from build123d import *

# Parameters (mm, degrees)
F0_R     = 3.175
F1_DEPTH = 25.4


with BuildPart() as f1:
    # F0 (on Top) → F1 (new body)
    with BuildSketch(Plane.XY):
        with BuildLine():
            ThreePointArc((9.4502929642, 115.490625), (0, 123.825), (-9.4502929642, 115.490625))
            ThreePointArc((-9.4502929642, 115.490625), (-7.14375, 107.9998046905), (0, 104.775))
            ThreePointArc((0, 104.775), (6.7351920908, 107.5648079092), (9.525, 114.3))
            ThreePointArc((9.525, 114.3), (9.5063048942, 114.896483242), (9.4502929642, 115.490625))
        make_face()
        with BuildLine():
            ThreePointArc((3.175, 114.3), (2.2450640303, 112.0549359697), (0, 111.125))
            ThreePointArc((0, 111.125), (-2.2450640303, 116.5450640303), (3.175, 114.3))
        make_face(mode=Mode.SUBTRACT)
        with BuildLine():
            Line((0, 100.0252), (0, 79.375))
            ThreePointArc((0, 79.375), (10.5003255158, 75.40625), (15.7504882737, 65.484375))
            Line((15.7504882737, 65.484375), (9.4502929642, 115.490625))
            ThreePointArc((9.4502929642, 115.490625), (9.5063048942, 114.896483242), (9.525, 114.3))
            ThreePointArc((9.525, 114.3), (6.7351920908, 107.5648079092), (0, 104.775))
            Line((0, 104.775), (0, 100.0252))
        make_face()
        with BuildLine():
            Line((-9.4502929642, 115.490625), (-15.7504882737, 65.484375))
            ThreePointArc((-15.7504882737, 65.484375), (-10.5003255158, 75.40625), (0, 79.375))
            Line((0, 79.375), (0, 100.0252))
            Line((0, 100.0252), (0, 104.775))
            ThreePointArc((0, 104.775), (-7.14375, 107.9998046905), (-9.4502929642, 115.490625))
        make_face()
        with Locations((-3.175, 100.0252)):
            Circle(F0_R, mode=Mode.SUBTRACT)
        with BuildLine():
            ThreePointArc((-9.4772553384, -0.9525), (-7.063929059, 6.3895642457), (0, 9.525))
            Line((0, 9.525), (0, 47.625))
            ThreePointArc((0, 47.625), (-10.6492737428, 51.7267849017), (-15.7954255641, 61.9125))
            Line((-15.7954255641, 61.9125), (-9.4772553384, -0.9525))
        make_face()
        with BuildLine():
            Line((0, 47.625), (0, 9.525))
            ThreePointArc((0, 9.525), (6.7351920908, 6.7351920908), (9.525, 0))
            Line((9.525, 0), (36.5125, 0))
            ThreePointArc((36.5125, 0), (38.9384772185, 5.7120069047), (44.7334821429, 7.9324362036))
            Line((44.7334821429, 7.9324362036), (18.9676000005, 8.8532337108))
            ThreePointArc((18.9676000005, 8.8532337108), (13.2611998974, 11.5713591498), (11.3411865923, 17.5933818124))
            Line((11.3411865923, 17.5933818124), (15.7954255641, 61.9125))
            ThreePointArc((15.7954255641, 61.9125), (10.6492737428, 51.7267849017), (0, 47.625))
        make_face()
        with BuildLine():
            Line((0, 60.325), (0, 47.625))
            ThreePointArc((0, 47.625), (10.6492737428, 51.7267849017), (15.7954255641, 61.9125))
            ThreePointArc((15.7954255641, 61.9125), (15.8550939106, 62.7052534459), (15.875, 63.5))
            ThreePointArc((15.875, 63.5), (15.8438414904, 64.4941387366), (15.7504882737, 65.484375))
            ThreePointArc((15.7504882737, 65.484375), (10.5003255158, 75.40625), (0, 79.375))
            Line((0, 79.375), (0, 66.675))
            ThreePointArc((0, 66.675), (2.2450640303, 65.7450640303), (3.175, 63.5))
            ThreePointArc((3.175, 63.5), (2.2450640303, 61.2549359697), (0, 60.325))
        make_face()
        with BuildLine():
            ThreePointArc((-15.7954255641, 61.9125), (-10.6492737428, 51.7267849017), (0, 47.625))
            Line((0, 47.625), (0, 60.325))
            ThreePointArc((0, 60.325), (-3.175, 63.5), (0, 66.675))
            Line((0, 66.675), (0, 79.375))
            ThreePointArc((0, 79.375), (-10.5003255158, 75.40625), (-15.7504882737, 65.484375))
            ThreePointArc((-15.7504882737, 65.484375), (-15.8737438155, 63.6997054867), (-15.7954255641, 61.9125))
        make_face()
        with BuildLine():
            Line((0, 9.525), (0, 3.175))
            ThreePointArc((0, 3.175), (2.2450640303, 2.2450640303), (3.175, 0))
            Line((3.175, 0), (9.525, 0))
            ThreePointArc((9.525, 0), (6.7351920908, 6.7351920908), (0, 9.525))
        make_face()
        with BuildLine():
            ThreePointArc((3.175, 0), (-2.2450640303, -2.2450640303), (0, 3.175))
            Line((0, 3.175), (0, 9.525))
            ThreePointArc((0, 9.525), (-7.063929059, 6.3895642457), (-9.4772553384, -0.9525))
            ThreePointArc((-9.4772553384, -0.9525), (-6.2623833816, -7.1769199091), (0.3401785714, -9.5189234444))
            ThreePointArc((0.3401785714, -9.5189234444), (6.8544082857, -6.6138273378), (9.525, 0))
            Line((9.525, 0), (3.175, 0))
        make_face()
        with BuildLine():
            Line((36.5125, 0), (9.525, 0))
            ThreePointArc((9.525, 0), (6.8544082857, -6.6138273378), (0.3401785714, -9.5189234444))
            Line((0.3401785714, -9.5189234444), (44.7334821429, -7.9324362036))
            ThreePointArc((44.7334821429, -7.9324362036), (38.9384772185, -5.7120069047), (36.5125, 0))
        make_face()
        with BuildLine():
            ThreePointArc((44.7334821429, 7.9324362036), (38.9384772185, 5.7120069047), (36.5125, 0))
            ThreePointArc((36.5125, 0), (38.9384772185, -5.7120069047), (44.7334821429, -7.9324362036))
            ThreePointArc((44.7334821429, -7.9324362036), (50.1620069047, -5.5115227815), (52.3875, 0))
            ThreePointArc((52.3875, 0), (50.1620069047, 5.5115227815), (44.7334821429, 7.9324362036))
        make_face()
        with BuildLine():
            ThreePointArc((47.625, 0), (44.45, -3.175), (41.275, 0))
            ThreePointArc((41.275, 0), (44.45, 3.175), (47.625, 0))
        make_face(mode=Mode.SUBTRACT)
    extrude(amount=F1_DEPTH)


solid = f1.part
Part model, mm, in its own coordinate system. A direction names the side the tool comes from. Coordinates: 2 decimals unless noted, no trailing zeros. Loops run counter-clockwise (first coordinate to the right, second up) from the corner with the lowest first, then second, coordinate; pieces in that order, holes last. Notation, with made-up numbers: (63, -16.5) -> (116, -16.5) arc R4 cw to (116, -9.5) -> close; hole circle Ø5 at (8.5, -39). An arc over 180 degrees is marked (long way). Use a Markdown table: item, result. Add a question column.
Item 1: Pull direction X, two halves, no side cores. Call faces 3 (the cylindrical face through (-3.588, 103.173, 12.522)), 4 (the cylindrical face through (41.52, -1.22, 12.52)), 5 (the cylindrical face through (-15.873, 63.725, 12.522)), 6 (the cylindrical face through (13.321, 11.503, 12.522)): +X half, -X half, draft (parallel to the pull), parting line (faces both ways), or undercut.
Item 2: Probe probe 1 along Y at (x, z) = (44.45, 10.75) (3 decimals); probe 2 along Y at (x, z) = (-4, 12); probe 3 along Y at (x, z) = (28.5, 2.75). List the from-to ranges inside material, lowest first.
Item 3: Flat gauge pins, fed straight in: P1, Ø5, axis at x = 22.5, z = 9.5, coming from the +Y side; P2, Ø6, axis at x = 1, z = 15.5, coming from the -Y side (3 decimals); P3, Ø1.5, axis at x = -7, z = 12.5, coming from the +Y side; P4, Ø3, axis at x = 24.5, z = 11, coming from the -Y side. Where does each tip first touch, or does it go through?
Item 4: Which spindle directions (+Z, -Z, +X, -X, +Y, -Y) get a long thin tool onto all of the face, cutting with end or side? Do faces 1 (the flat face through (13.537, 39.443, 12.522)), 2 (the flat face through (-12.68, 30.92, 12.52)). Say none if no direction does.
Item 5: Band-saw the part on C-C on y = 86.5. Write the cut outline in (x, z), plus the area to 3 significant figures.
Item 6: Band-saw the part on D-D on x = 7. Write the cut outline in (y, z).
Item 7: Band-saw the part on A-A on x = -1.5. Write the cut outline in (y, z).
Item 8: Band-saw the part on B-B on z = 2.5. Give the number of separate pieces and of enclosed holes in the cut face, plus the area to 3 significant figures.
Geometry says:
| question | item | result |
|---|---|---|
| 1 | face 3 | undercut |
| 1 | face 4 | undercut |
| 1 | face 5 | -X half |
| 1 | face 6 | +X half |
| 2 | probe 1 | -7.943 to -3.175, 3.175 to 7.943 |
| 2 | probe 2 | -8.64 to 96.96, 103.09 to 122.94 |
| 2 | probe 3 | -8.51 to 8.51 |
| 3 | P1 | y = 8.82 |
| 3 | P2 | y = -9.525 |
| 3 | P3 | y = 121.49 |
| 3 | P4 | y = -8.71 |
| 4 | face 1 | +Z, -Z, +X |
| 4 | face 2 | +Z, -Z, -X, -Y |
| 5 | outline | (-13.1, 0) -> (13.1, 0) -> (13.1, 25.4) -> (-13.1, 25.4) -> close |
| 5 | area | 666 mm² |
| 6 | outline | (-9.28, 0) -> (120.76, 0) -> (120.76, 25.4) -> (-9.28, 25.4) -> close |
| 7 | outline | (-9.41, 0) -> (-2.8, 0) -> (-2.8, 25.4) -> (-9.41, 25.4) -> close; (2.8, 0) -> (60.7, 0) -> (60.7, 25.4) -> (2.8, 25.4) -> close; (66.3, 0) -> (97.33, 0) -> (97.33, 25.4) -> (66.3, 25.4) -> close; (102.72, 0) -> (111.5, 0) -> (111.5, 25.4) -> (102.72, 25.4) -> close; (117.1, 0) -> (123.71, 0) -> (123.71, 25.4) -> (117.1, 25.4) -> close |
| 8 | separate pieces | 1 |
| 8 | enclosed holes | 5 |
| 8 | area | 3,770 mm² |
